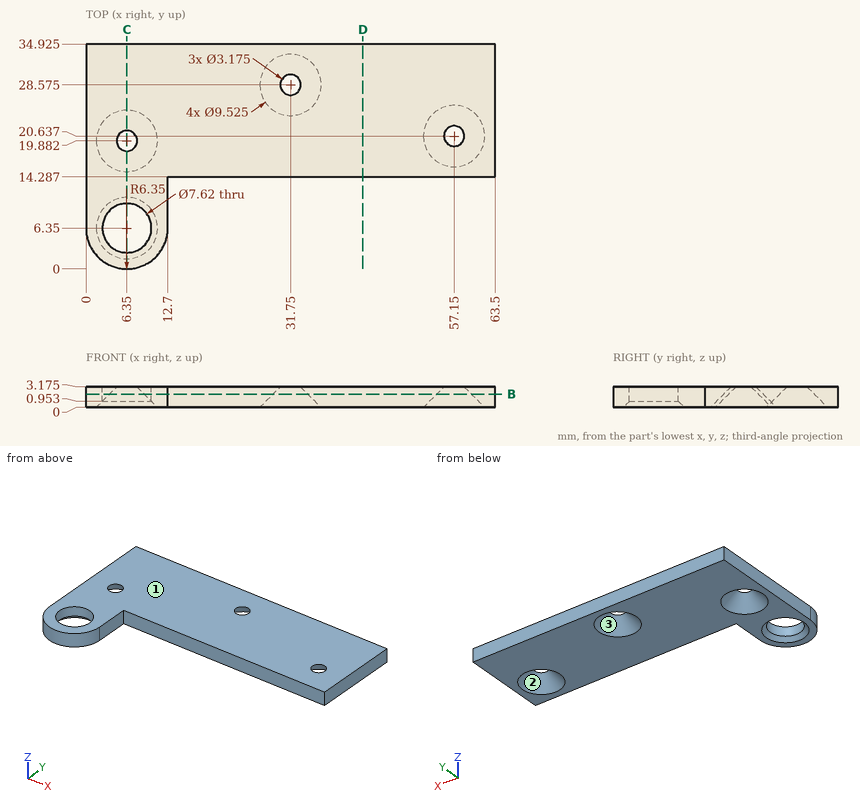
Job drawing, mm, ordinate dimensions from the low corner. One solid piece. Give positions to 0.01 mm unless a question says otherwise; leave off trailing zeros. Write each loop counter-clockwise with the first axis right and the second up, starting at its lowest first coordinate (ties: lowest second). Pieces come first, ordered by that corner, then holes. Notation, with made-up numbers: M 72.5,-33 L 98.5,-33 A15 ccw 98.5,-22 Z; hole C 39.25,23.5 d5. An arc over 180 degrees is marked long. Put each result on its own line as item: value. Start each with the question number.
(1) Mould opens along X. For the marked faces 1, 2 and 3 say: +X half, -X half, draft (parallel to the pull), parting line (faces both ways), or undercut.
(2) Flat gauge pins, fed straight in: pin 1 Ø1.6 at (y, z) = (9, 2) entering from +X; pin 2 Ø4.5 at (x, y) = (6.35, 6.35) entering from +Z; pin 3 Ø1 at (x, z) = (31.5, 1.5) entering from -Y. Where does each tip first touch, or does it go through?
(3) Band-saw the part on C-C, the plane x = 6.35. Write the cut outline in (y, z) (1 decimal).
(4) Probe L1, parallel to X at y = 6.35, z = 1.6; L2, parallel to Y at x = 6.35, z = 2.45 (1 decimal); L3, parallel to Y at x = 6.35, z = 2.7 (1 decimal). List the from-to ranges inside material, lowest first.
(5) Band-saw the part on D-D, the plane x = 43. Write the cut outline in (y, z) (1 decimal).
(6) Band-saw the part on B-B, the plane z = 2.05. Give the number of separate pieces and of enclosed holes in the cut face, and give its area (3 significant figures).
Response values:
1. face 1: draft
1. face 2: undercut
1. face 3: undercut
2. pin 1: stops at x = 12.7
2. pin 2: passes through
2. pin 3: stops at y = 14.29
3. outline: M 0,0 L 1.6,0 L 2.5,1 L 2.5,3.2 L 0,3.2 Z; M 10.2,1 L 11.1,0 L 15.1,0 L 18.3,3.2 L 10.2,3.2 Z; M 21.5,3.2 L 24.6,0 L 34.9,0 L 34.9,3.2 Z
4. L1: x = 0 to 2.54, 10.16 to 12.7
4. L2: y = 0 to 2.5, 10.2 to 17.6, 22.2 to 34.9
4. L3: y = 0 to 2.5, 10.2 to 17.8, 21.9 to 34.9
5. outline: M 14.3,0 L 34.9,0 L 34.9,3.2 L 14.3,3.2 Z
6. separate pieces: 1
6. enclosed holes: 4
6. area: 1,360 mm2
